Design review of the part built by this model. Coordinates are the model's own, in mm. A direction names the side the tool comes from. Coordinates: 2 decimals unless noted, no trailing zeros. Loops run counter-clockwise (first coordinate to the right, second up) from the corner with the lowest first, then second, coordinate; pieces in that order, holes last. Notation, with made-up numbers: M 21.25,89.5 L 29.25,89.5 A29 cw 29.25,125.5 Z; hole C -26,5 d1. An arc over 180 degrees is marked long. Answer as a JSON object with one key per item and string values. Group by question number.
1. Consider section B-B (x = 0). State the section outline as (y, z) points.
2. Consider section A-A (y = 0). State the section outline as (x, z) points.
3. Draft analysis for pull direction X (two halves, no side actions). For faces 1 (the cylindrical face through (0, -2, 4)), 2 (the cylindrical face through (4.516, -0.421, 1.369)), 3 (the flat face through (1, 1, 6)), state which applies: +X half, -X half, draft (parallel to the pull), parting line (faces both ways), or undercut.
4. Insertion check: pin 1 (2.5 mm diameter, centred on x = -3.5, y = 0, fed in from +Z); pin 2 (1 mm diameter, centred on y = 4, z = 3, fed in from -X). Each pin has a flat end and moves straight along its axis. Give the tip position at first contact, or say it passes through.
5. Consider section C-C (z = 4). State the section outline as (x, y) points.
6. Machinability: for faces 4 (the flat face through (2.2, 0.1, 2.7)), 5 (the cylindrical face through (-0.27, -1.22, 3.04)), which of the approach directions +Z, -Z, +X, -X, +Y, -Y give a long, thin tool a straight path to every point of the face, cutting with its end or side? Answer none if there is none.
7. Consider section D-D (x = 2.75). State the section outline as (y, z) points, then the cut area to 3 significant figures.
8. To check wall thickness, follow probe 1 along Z at (x, y) = (-0.25, 3.75); probe 2 along Y at (x, z) = (3.5, 1.85); probe 3 along Y at (x, z) = (-0.5, 1.25). State the ranges of each line that lie inside material, in increasing order.
Autodesk Inventor part; units mm, degrees
ref_plane "YZ Plane" through (0, 0, 0) normal (1, 0, 0) x (0, 1, 0)
ref_plane "XZ Plane" through (0, 0, 0) normal (0, 1, 0) x (-1, 0, 0)
ref_plane "XY Plane" through (0, 0, 0) normal (0, 0, 1) x (1, 0, 0)
sketch "スケッチ1" plane through (0, 0, 0) normal (0, 0, 1) x (1, 0, 0)
  circle A0 centre (0, 0) radius 5
  dimension "d0" = 10
extrude "押し出し1" add sketch "スケッチ1" along normal blind 6
sketch "スケッチ2" plane through (0, 0, 6) normal (0, 0, 1) x (1, 0, 0)
  circle A0 centre (0, 0) radius 5
  circle A1 centre (0, 0) radius 2
  dimension "d3" = 4
extrude "押し出し2" cut sketch "スケッチ2" against normal blind 3.3
sketch "スケッチ3" plane through (0, 0, 6) normal (0, 0, 1) x (1, 0, 0)
  circle A0 centre (0, 0) radius 1.25
  dimension "d6" = 2.5
extrude "押し出し3" cut sketch "スケッチ3" against normal blind 6
sketch "スケッチ4" plane through (0, 0, 2.7) normal (0, 0, 1) x (1, 0, 0)
  circle A0 centre (0, 0) radius 3.5
  circle A1 centre (-3.5, 0) radius 1.1
  circle A2 centre (3.5, 0) radius 1.1
  dimension "d9" = 7
  dimension "d10" = 2.2
  dimension "d11" = 2.2
extrude "押し出し4" cut sketch "スケッチ4" against normal blind 6 contours A0 A2 | A0 A2 | A1 A0 | A0 A1
properties part number "homemade_setcolor-2_jig"
Findings below:
{
 "1": {"outline": "M -5,0 L -1.25,0 L -1.25,6 L -2,6 L -2,2.7 L -5,2.7 Z; M 1.25,0 L 5,0 L 5,2.7 L 2,2.7 L 2,6 L 1.25,6 Z"},
 "2": {"outline": "M -5,0 L -4.6,0 L -4.6,2.7 L -5,2.7 Z; M -2.4,0 L -1.25,0 L -1.25,6 L -2,6 L -2,2.7 L -2.4,2.7 Z; M 1.25,0 L 2.4,0 L 2.4,2.7 L 2,2.7 L 2,6 L 1.25,6 Z; M 4.6,0 L 5,0 L 5,2.7 L 4.6,2.7 Z"},
 "3": {"face 1": "parting line", "face 2": "undercut", "face 3": "draft"},
 "4": {"pin 1": "stops at z = 2.7", "pin 2": "stops at x = -3.47"},
 "5": {"outline": "C 0,0 d4; hole C 0,0 d2.5"},
 "6": {"face 4": "+Z", "face 5": "+Z, -Z"},
 "7": {"outline": "M -4.18,0 L -0.8,0 L -0.8,2.7 L -4.18,2.7 Z; M 0.8,0 L 4.18,0 L 4.18,2.7 L 0.8,2.7 Z", "area": "18.2 mm^2"},
 "8": {"probe 1": "z = 0 to 2.7", "probe 2": "y = -3.57 to -1.1, 1.1 to 3.57", "probe 3": "y = -4.97 to -1.15, 1.15 to 4.97"}
}
